```python
from build123d import *

# Parameters (mm, degrees)
BOSS_EXTRUDE1_DEPTH   = 1.27
SKETCH1_W             = 3.3528
SKETCH1_H             = 2.50444
BOSS_EXTRUDE1_2_DEPTH = 1.27
FILLET3_R             = 0.8128
FILLET4_R             = 0.8128
SKETCH5_W             = 2.54
SKETCH5_H             = 5.00888
BOSS_EXTRUDE3_DEPTH   = 5.08
SKETCH6_W             = 19.05
SKETCH6_H             = 19.05
SKETCH6_W_2           = 13.97
SKETCH6_H_2           = 13.97
BOSS_EXTRUDE4_DEPTH   = 3.175
SKETCH7_W             = 2.54
SKETCH7_H             = 1.778
SKETCH7_W_2           = 1.778
SKETCH7_H_2           = 2.54
CUT_EXTRUDE2_DEPTH    = 1.778
FILLET6_R             = 0.889


with BuildPart() as part:
    # Sketch1 → Boss-Extrude1 (new body)
    with BuildSketch(Plane(origin=(0, 0, 0), x_dir=(1, 0, 0), z_dir=(0, 1, 0))):
        Polygon((0.8128, 1.061632718), (0.8128, -0.370927282), (5.29336, -0.370927282), (5.29336, 0.441872718), (7.7978, 0.441872718), (7.7978, -2.910927282), (-1.7272, -2.910927282), (-1.7272, 1.061632718), align=None)
    extrude(amount=BOSS_EXTRUDE1_DEPTH)

    # Fillet3
    fillet3_edges = [part.edges().sort_by_distance(p)[0] for p in [
        (6.54558, 1.27, -0.441872718),
    ]]
    fillet(fillet3_edges, radius=FILLET3_R)


with BuildPart() as body_2:
    # Sketch1 → Boss-Extrude1 2 (new body)
    with BuildSketch(Plane(origin=(0, 0, 0), x_dir=(1, 0, 0), z_dir=(0, 1, 0))):
        with Locations((-0.0508, 5.361852718)):
            Rectangle(SKETCH1_W, SKETCH1_H)
    extrude(amount=BOSS_EXTRUDE1_2_DEPTH)

    # Fillet4
    fillet4_edges = [body_2.edges().sort_by_distance(p)[0] for p in [
        (1.6256, 1.27, -5.361852718),
    ]]
    fillet(fillet4_edges, radius=FILLET4_R)


with BuildPart() as body_3:
    # Mirror6: mirrored copy
    add(part.part.mirror(Plane(origin=(7.7978, 1.27, -0.441872718), x_dir=(0, 0, 1), z_dir=(-1, 0, 0))))


with BuildPart() as body_4:
    # Mirror6 2: mirrored copy
    add(body_2.part.mirror(Plane(origin=(7.7978, 1.27, -0.441872718), x_dir=(0, 0, 1), z_dir=(-1, 0, 0))))


with BuildPart() as body_5:
    # Mirror7: mirrored copy
    add(body_3.part.mirror(Plane(origin=(17.3228, 1.27, -6.614072718), x_dir=(1, 0, 0), z_dir=(0, 0, 1))))


with BuildPart() as body_6:
    # Mirror7 2: mirrored copy
    add(body_4.part.mirror(Plane(origin=(17.3228, 1.27, -6.614072718), x_dir=(1, 0, 0), z_dir=(0, 0, 1))))


with BuildPart() as body_7:
    # Mirror8: mirrored copy
    add(body_5.part.mirror(Plane(origin=(7.7978, 1.27, -12.786272718), x_dir=(0, 0, 1), z_dir=(1, 0, 0))))


with BuildPart() as body_8:
    # Mirror8 2: mirrored copy
    add(body_6.part.mirror(Plane(origin=(7.7978, 1.27, -12.786272718), x_dir=(0, 0, 1), z_dir=(1, 0, 0))))


with BuildPart() as part_1:
    add(part.part)

    add(body_2.part)  # Boss-Extrude3 merges body 2

    add(body_3.part)  # Boss-Extrude3 merges body 3

    add(body_4.part)  # Boss-Extrude3 merges body 4

    add(body_5.part)  # Boss-Extrude3 merges body 5

    add(body_6.part)  # Boss-Extrude3 merges body 6

    add(body_7.part)  # Boss-Extrude3 merges body 7

    add(body_8.part)  # Boss-Extrude3 merges body 8
    # Sketch5 → Boss-Extrude3 (add)
    with BuildSketch(Plane.XZ):
        Polygon((17.3228, -1.061632718), (14.7828, -1.061632718), (14.7828, 0.370927282), (0.8128, 0.370927282), (0.8128, -1.061632718), (-1.7272, -1.061632718), (-1.7272, 2.910927282), (17.3228, 2.910927282), align=None)
        Polygon((17.3228, -16.139072718), (-1.7272, -16.139072718), (-1.7272, -12.166512718), (0.8128, -12.166512718), (0.8128, -13.599072718), (14.7828, -13.599072718), (14.7828, -12.166512718), (17.3228, -12.166512718), align=None)
        with Locations((16.0528, -6.614072718)):
            Rectangle(SKETCH5_W, SKETCH5_H)
        with Locations((-0.4572, -6.614072718)):
            Rectangle(SKETCH5_W, SKETCH5_H)
    extrude(amount=BOSS_EXTRUDE3_DEPTH)

    # Sketch6 → Boss-Extrude4 (add)
    with BuildSketch(Plane.XZ.offset(5.08)):
        with Locations((7.7978, -6.614072718)):
            Rectangle(SKETCH6_W, SKETCH6_H)
        with Locations((7.7978, -6.614072718)):
            Rectangle(SKETCH6_W_2, SKETCH6_H_2, mode=Mode.SUBTRACT)
    extrude(amount=BOSS_EXTRUDE4_DEPTH)

    # Sketch7 → Cut-Extrude2 (cut)
    with BuildSketch(Plane.XZ.offset(8.255)):
        with Locations((-0.4572, -5.598072718)):
            Rectangle(SKETCH7_W, SKETCH7_H)
        with Locations((-0.4572, -3.058072718)):
            Rectangle(SKETCH7_W, SKETCH7_H)
        with Locations((10.5918, 1.640927282)):
            Rectangle(SKETCH7_W_2, SKETCH7_H_2)
        with Locations((5.0038, 1.640927282)):
            Rectangle(SKETCH7_W_2, SKETCH7_H_2)
        with Locations((10.5918, -14.869072718)):
            Rectangle(SKETCH7_W_2, SKETCH7_H_2)
        with Locations((5.0038, -14.869072718)):
            Rectangle(SKETCH7_W_2, SKETCH7_H_2)
        with Locations((16.0528, -5.598072718)):
            Rectangle(SKETCH7_W, SKETCH7_H)
        with Locations((16.0528, -3.058072718)):
            Rectangle(SKETCH7_W, SKETCH7_H)
    extrude(amount=-CUT_EXTRUDE2_DEPTH, mode=Mode.SUBTRACT)

    # Fillet6
    fillet6_edges = [part_1.edges().sort_by_distance(p)[0] for p in [
        (-0.4572, -6.477, -4.709072718),
        (16.0528, -6.477, -4.709072718),
        (11.4808, -6.477, 1.640927282),
        (5.8928, -6.477, 1.640927282),
        (9.7028, -6.477, 1.640927282),
        (4.1148, -6.477, 1.640927282),
        (-0.4572, -6.477, -2.169072718),
        (16.0528, -6.477, -2.169072718),
        (-0.4572, -6.477, -6.487072718),
        (-0.4572, -6.477, -3.947072718),
        (16.0528, -6.477, -3.947072718),
        (16.0528, -6.477, -6.487072718),
        (4.1148, -6.477, -14.869072718),
        (9.7028, -6.477, -14.869072718),
        (5.8928, -6.477, -14.869072718),
        (11.4808, -6.477, -14.869072718),
    ]]
    fillet(fillet6_edges, radius=FILLET6_R - 0.0001)  # a hair under: the kernel refuses the full size


solid = part_1.part
```
Could you check a few things on this model? Use its own coordinates, in mm. A direction names the side the tool comes from. Round coordinates to 2 decimals unless told otherwise and drop trailing zeros. Loops run counter-clockwise (first coordinate to the right, second up) from the corner with the lowest first, then second, coordinate; pieces in that order, holes last. Notation, with made-up numbers: (68.5, -33.5) - (82.5, -33.5) arc R19 cw to (82.5, -4.5) - close; hole circle Ø9 at (64, 18). An arc over 180 degrees is marked (long way). Answer in a Markdown table with one row per item. Add a question column.
(1) If we section it at C-C (y = -2): Please give me the cut outline in (x, z).
(2) I need wall thicknesses on line 1 along Z through (x, y) = (-0.75, -0.5); line 2 along Z through (x, y) = (5.75, -4.5); line 3 along X through (y, z) = (-4.25, 0). Which ranges of each line are inside material? Lowest first, please.
(3) If we section it at D-D (x = 14.5): Please give me the cut outline in (y, z) (3 decimals).
(4) For faces 3 (the face through (16, -8, -6.487)), 4 (the face through (11.481, -8, 2)), 5 (the face through (0, -2, -1.062)), which set-ups out of +Z, -Z, +X, -X, +Y, -Y let a thin tool reach every point of the face, with its end or its side?
(5) I'm going to push a flat-ended pin straight in: pin 1 (1.3 mm diameter, centred on x = 16.5, z = -2.5, fed in from +Y). Where does the tip first touch, or does it pass through?
(6) If we section it at A-A (x = 8.5): Please give me the cut outline in (y, z) (3 decimals), plus the area to 3 significant figures.
(7) If we mould it in two halves opening along X, with no side actions, what happens to faces 1 (the face through (10.302, 0.6, -13.2)), 2 (the face through (16, -8, -2.169))? For each: pulls with the +X half, pulls with the -X half, needs draft (parallel to the pull), parting line crosses it, or undercut.
(8) If we section it at B-B (z = -8.25): Please give me the cut outline in (x, y) (3 decimals).
Model answer:
| question | item | result |
|---|---|---|
| 1 | outline | (-1.73, -16.14) - (17.32, -16.14) - (17.32, -12.17) - (14.78, -12.17) - (14.78, -13.6) - (0.81, -13.6) - (0.81, -12.17) - (-1.73, -12.17) - close; (-1.73, -9.12) - (0.81, -9.12) - (0.81, -4.11) - (-1.73, -4.11) - close; (-1.73, -1.06) - (0.81, -1.06) - (0.81, 0.37) - (14.78, 0.37) - (14.78, -1.06) - (17.32, -1.06) - (17.32, 2.91) - (-1.73, 2.91) - close; (14.78, -9.12) - (17.32, -9.12) - (17.32, -4.11) - (14.78, -4.11) - close |
| 2 | line 1 | z = -16.14 to -12.17, -9.12 to -4.11, -1.06 to 2.91 |
| 2 | line 2 | z = -16.14 to -13.6, 0.37 to 2.91 |
| 2 | line 3 | x = -1.73 to 0.81, 14.78 to 17.32 |
| 3 | outline | (-8.255, -16.139) - (1.27, -16.139) - (1.27, -13.599) - (-8.255, -13.599) - close; (-8.255, 0.371) - (1.27, 0.371) - (1.27, 2.911) - (-8.255, 2.911) - close; (0, -9.119) - (1.219, -9.119) - (1.219, -4.11) - (0, -4.11) - close |
| 4 | face 3 | +X, -X, -Y |
| 4 | face 4 | +Z, -Z, -Y |
| 4 | face 5 | +X, -X, +Y |
| 5 | pin 1 | stops at y = -5.08 |
| 6 | outline | (-8.255, -16.139) - (1.27, -16.139) - (1.27, -13.599) arc R0.813 ccw to (0.457, -12.786) - (0, -12.786) - (0, -13.599) - (-8.255, -13.599) - close; (-8.255, 0.371) - (0, 0.371) - (0, -0.442) - (0.457, -0.442) arc R0.813 ccw to (1.27, 0.371) - (1.27, 2.911) - (-8.255, 2.911) - close |
| 6 | area | 50.2 mm² |
| 7 | face 1 | undercut |
| 7 | face 2 | needs draft |
| 8 | outline | (-1.727, -8.255) - (0.813, -8.255) - (0.813, 0) - (1.626, 0) - (1.626, 0.457) arc R0.813 ccw to (0.813, 1.27) - (-1.727, 1.27) - close; (13.97, 0) - (14.783, 0) - (14.783, -8.255) - (17.323, -8.255) - (17.323, 1.27) - (14.783, 1.27) arc R0.813 ccw to (13.97, 0.457) - close |
